Source: CAD feature listing. Evaluate the final solid. Frame: model axes, mm. Coordinates: 2 decimals unless noted, no trailing zeros. Loops run counter-clockwise (first coordinate to the right, second up) from the corner with the lowest first, then second, coordinate; pieces in that order, holes last.
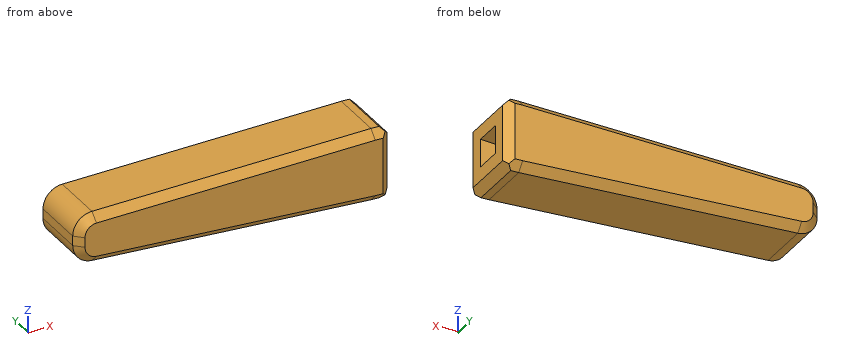
Autodesk Fusion 360 part; units mm, degrees
sketch "Sketch1" plane through (0, 0, 0) normal (0, 1, 0) x (1, 0, 0)
  line L0 (0, 0) -> (-78.5, 0)
  line L1 (-78.5, 0) -> (-78.5, 18)
  line L2 (-78.5, 18) -> (0, 18)
  line L3 (0, 18) -> (0, 0)
  line L4 (-4, 18) -> (-78.5, 15)
  line L5 (-4, 0) -> (-78.5, 3)
  dimension "d1" = 78.5
  dimension "d2" = 18
  dimension "d3" = 4
  dimension "d4" = 3
  dimension "d5" = 3
extrude "Extrude1" add sketch "Sketch1" along normal blind 18 contours L0 L1 L2 L3 L4 L5
sketch "Sketch2" plane through (0, 0, 0) normal (1, 0, 0) x (0, 0, -1)
  line L0 (0, 0) -> (18, 0)
  line L1 (18, 0) -> (18, 18)
  line L2 (18, 18) -> (0, 18)
  line L3 (0, 18) -> (0, 0)
  line L4 (18, 18) -> (0, 0) construction
  line L5 (12.5, 5.5) -> (5.5, 5.5)
  line L6 (5.5, 5.5) -> (5.5, 12.5)
  line L7 (5.5, 12.5) -> (12.5, 12.5)
  line L8 (12.5, 12.5) -> (12.5, 5.5)
  line L9 (12.5, 5.5) -> (5.5, 12.5) construction
  line L10 (5.5, 5.5) -> (12.5, 12.5) construction
  point P0 (9, 9)
  dimension "d8" = 7
  dimension "d9" = 7
extrude "Extrude2" cut sketch "Sketch2" against normal blind 15 contours L5 L6 L7 L8
chamfer "Chamfer1" distance 2 angle 45 4 edges at (0, 18, -9) (0, 9, -18) (0, 9, 0) (0, 0, -9)
fillet "Fillet1" radius 5 2 edges at (-78.5, 9, -3) (-78.5, 9, -15)
chamfer "Chamfer3" distance 2 angle 45 14 edges at (-38.8506, 18, -1.4034) (-38.8506, 18, -16.5966) (-77.106, 18, -13.661) (-78.5, 18, -9) (-77.106, 18, -4.339) (-3, 18, -18) (-3, 18, 0) (-38.8506, 0, -1.4034) (-77.106, 0, -4.339) (-78.5, 0, -9) (-77.106, 0, -13.661) (-38.8506, 0, -16.5966) (-3, 0, -18) (-3, 0, 0)
chamfer "Chamfer4" distance 15 distance2 1 2 edges at (-15, 9, -12.5) (-15, 9, -5.5) measured on face at (-5, 10.1667, -12.5) measured on face at (-5, 7.8333, -5.5)
equation "d8 = Switch_Thickness"
equation "d9 = Switch_Thickness"
equation "Switch_Thickness = 7 mm"
Q1. Section C-C, the plane z = -9.25. Return the cut outline in (x, y), plus the area to 3 significant figures.
Q2. Contact query for flat-ended pins moving along their axis: pin 1 Ø3 at (y, z) = (3.5, -3.5) entering from -X; pin 2 Ø1 at (y, z) = (10, -11.5) entering from -X; pin 3 Ø8 at (x, y) = (-37, 15) entering from +Z; pin 4 Ø10 at (x, z) = (-59.5, -11) entering from -Y. Output: stop coordinate, or through.
Q3. Line query: line 1 along Z through (x, y) = (-27.5, 15.75); line 2 along Y through (x, z) = (-28.5, -2); line 3 along Z through (x, y) = (-36, 10). Output: solid intervals per line, ascending.
Q4. Section B-B, the plane x = -39. Return the cut outline in (y, z), plus the area to 3 significant figures.
Q5. Section D-D, the plane x = -5. Return the cut outline in (y, z).
Derived:
1. outline: (-78.5, 2) - (-76.5, 0) - (-2, 0) - (0, 2) - (0, 5.5) - (-15, 5.5) - (-15, 12.5) - (0, 12.5) - (0, 16) - (-2, 18) - (-76.5, 18) - (-78.5, 16) - close
1. area: 1,300 mm2
2. pin 1: stops at x = -77.64
2. pin 2: stops at x = -78.44
2. pin 3: stops at z = -1.17
2. pin 4: stops at y = 0
3. line 1: z = -17.05 to -0.95
3. line 2: y = 0.99 to 17.01
3. line 3: z = -16.71 to -1.29
4. outline: (0, -14.59) - (2, -16.59) - (16, -16.59) - (18, -14.59) - (18, -3.41) - (16, -1.41) - (2, -1.41) - (0, -3.41) - close
4. area: 265 mm2
5. outline: (0, -15.96) - (2, -17.96) - (16, -17.96) - (18, -15.96) - (18, -2.04) - (16, -0.04) - (2, -0.04) - (0, -2.04) - close; hole (5.5, -12.17) - (12.5, -12.17) - (12.5, -5.83) - (5.5, -5.83) - close
